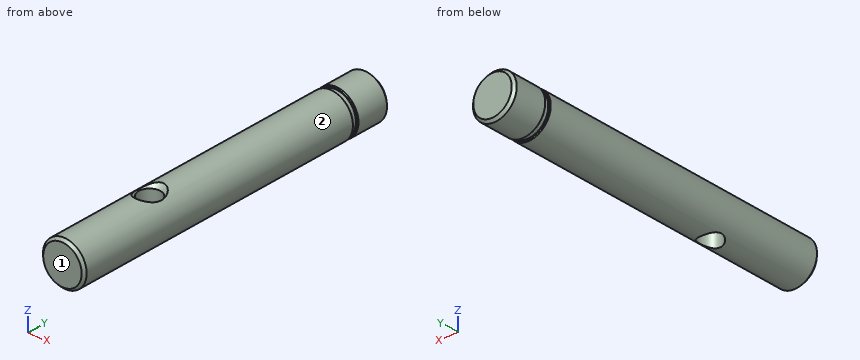
```python
from build123d import *

# Parameters (mm, degrees)
F0_R           = 2.5
F0_R_2         = 2.3
F1_DEPTH       = 38.5
F2_SIZE        = 0.3
F5_D           = 2.5
F5_CSINK_D     = 4.5
F5_CSINK_ANGLE = 90
F6_START       = 4
F6_DEPTH       = 0.5
F7_SIZE        = 0.1


with BuildPart() as f1:
    # F0 (on Front) → F1 (new body)
    with BuildSketch(Plane.XZ):
        Circle(F0_R)
        Circle(F0_R_2, mode=Mode.SUBTRACT)
        Circle(F0_R_2)
    extrude(amount=F1_DEPTH)

    # F2
    f2_edges = [f1.edges().sort_by_distance(p)[0] for p in [
        (-2.5, -38.5, 0),
        (-2.5, 0, 0),
    ]]
    chamfer(f2_edges, length=F2_SIZE)

    # F5 (through all)
    with Locations(Plane.XY.offset(3)):
        with Locations((0, -27.5)):
            CounterSinkHole(F5_D / 2, F5_CSINK_D / 2, counter_sink_angle=F5_CSINK_ANGLE)

    # F0 (on Front) → F6 (cut)
    with BuildSketch(Plane.XZ.offset(F6_START)):
        Circle(F0_R)
        Circle(F0_R_2, mode=Mode.SUBTRACT)
    extrude(amount=F6_DEPTH, mode=Mode.SUBTRACT)

    # F7
    f7_edges = [f1.edges().sort_by_distance(p)[0] for p in [
        (-2.5, -4, 0),
        (-2.5, -4.5, 0),
    ]]
    chamfer(f7_edges, length=F7_SIZE)


solid = f1.part
```
The model under review builds one solid part; all positions refer to its coordinate system, in mm. Face numbers are marked on the shaded views. Round coordinates to 2 decimals unless told otherwise and drop trailing zeros. Order: outer loops, then holes, each group sorted by start corner. A loop starts at its lowest first (then second) coordinate and runs counter-clockwise, first axis right, second up. Notation, with made-up numbers: (-23.75, -12.5) -> (10.25, -12.5) arc R30 ccw to (10.25, 23.5) -> close; hole circle Ø11 at (-11, -22.5). An arc over 180 degrees is marked (long way). Use a Markdown table: item, result.
Q1. Mouldability with a two-part tool opening along X and no side actions: class the marked faces 1 and 2 as +X half, -X half, draft (parallel to the pull), parting line (faces both ways), or undercut.
Values:
| item | result |
|---|---|
| face 1 | draft |
| face 2 | parting line |
Q2. Clearance check with a flat-ended pin moving along its axis: P1, Ø1.5, axis at x = -1.5, y = -7, coming from the +Z side. State where the tip first meets the part, or that it passes through.
Values:
| item | result |
|---|---|
| P1 | stops at z = 2.38 |
Q3. We need section C-C on y = -27.5. Write out the cut boundary in (x, z), then the cut area to 3 significant figures.
Values:
| item | result |
|---|---|
| outline | (-1.35, 2.1) arc R2.5 ccw to (-1.25, -2.17) -> (-1.25, 2) -> close; (1.25, -2.17) arc R2.5 ccw to (1.35, 2.1) -> (1.25, 2) -> close |
| area | 7.66 mm^2 |
Q4. We need section D-D on y = -21. Write out the cut boundary in (x, z), then the cut area to 3 significant figures.
Values:
| item | result |
|---|---|
| outline | circle Ø5 at (0, 0) |
| area | 19.6 mm^2 |
Q5. We need section B-B on x = 0. Write out the cut boundary in (y, z), then the cut area to 3 significant figures.
Values:
| item | result |
|---|---|
| outline | (-38.5, -2.2) -> (-38.2, -2.5) -> (-28.75, -2.5) -> (-28.75, 2) -> (-29.25, 2.5) -> (-38.2, 2.5) -> (-38.5, 2.2) -> close; (-26.25, -2.5) -> (-4.6, -2.5) -> (-4.5, -2.4) -> (-4.5, -2.3) -> (-4, -2.3) -> (-4, -2.4) -> (-3.9, -2.5) -> (-0.3, -2.5) -> (0, -2.2) -> (0, 2.2) -> (-0.3, 2.5) -> (-3.9, 2.5) -> (-4, 2.4) -> (-4, 2.3) -> (-4.5, 2.3) -> (-4.5, 2.4) -> (-4.6, 2.5) -> (-25.75, 2.5) -> (-26.25, 2) -> close |
| area | 179 mm^2 |
Q6. For line 1 (Y direction, x = 0, z = 0.9); line 2 (X direction, y = -27.5, z = 0.2); line 3 (X direction, y = -27.5, z = -0.7), list the stretches that pass through material, from the lowest coordinate up.
Values:
| item | result |
|---|---|
| line 1 | y = -38.5 to -28.75, -26.25 to 0 |
| line 2 | x = -2.49 to -1.25, 1.25 to 2.49 |
| line 3 | x = -2.4 to -1.25, 1.25 to 2.4 |
Q7. We need section A-A on z = 0. Write out the cut boundary in (x, y), then the cut area to 3 significant figures.
Values:
| item | result |
|---|---|
| outline | (-2.5, -38.2) -> (-2.2, -38.5) -> (2.2, -38.5) -> (2.5, -38.2) -> (2.5, -4.6) -> (2.4, -4.5) -> (2.3, -4.5) -> (2.3, -4) -> (2.4, -4) -> (2.5, -3.9) -> (2.5, -0.3) -> (2.2, 0) -> (-2.2, 0) -> (-2.5, -0.3) -> (-2.5, -3.9) -> (-2.4, -4) -> (-2.3, -4) -> (-2.3, -4.5) -> (-2.4, -4.5) -> (-2.5, -4.6) -> close; hole circle Ø2.5 at (0, -27.5) |
| area | 187 mm^2 |
